from build123d import *

# Parameters (mm, degrees)
F0_R     = 3.5
F0_R_2   = 1.925
F1_DEPTH = 3.9
F2_DEPTH = 10
F4_DEPTH = 2
F5_R     = 0.25


with BuildPart() as f1:
    # F0 (on Front) → F1 (new body)
    with BuildSketch(Plane.XZ):
        Circle(F0_R)
        Circle(F0_R_2, mode=Mode.SUBTRACT)
        Circle(F0_R_2)
    extrude(amount=F1_DEPTH)

    # F0 (on Front) → F2 (join)
    with BuildSketch(Plane.XZ):
        Circle(F0_R_2)
    extrude(amount=-F2_DEPTH)

    # F3 (on face) → F4 (cut)
    with BuildSketch(Plane.XZ.offset(3.9)):
        Polygon((1.5, -0.8660254038), (1.5, 0.8660254038), (0, 1.7320508076), (-1.5, 0.8660254038), (-1.5, -0.8660254038), (0, -1.7320508076), align=None)
    extrude(amount=-F4_DEPTH, mode=Mode.SUBTRACT)

    # F5
    f5_edges = [f1.edges().sort_by_distance(p)[0] for p in [
        (-3.5, -3.9, 0),
    ]]
    fillet(f5_edges, radius=F5_R)


solid = f1.part
Read the model definition and answer for the solid it produces. Units are mm, in the model's axes. A direction names the side the tool comes from. Give positions to 0.01 mm unless a question says otherwise; leave off trailing zeros. Write each loop counter-clockwise with the first axis right and the second up, starting at its lowest first coordinate (ties: lowest second). Pieces come first, ordered by that corner, then holes. Notation, with made-up numbers: (66.5, -15) - (115.5, -15) arc R27 cw to (115.5, 23) - close; hole circle Ø7 at (-33.75, -31). An arc over 180 degrees is marked (long way). Answer in a Markdown table with one row per item. Add a question column.
Item 1: Section B-B, the plane z = 0 is taken. Write down the section's boundary in (x, y) (3 decimals).
Item 2: Section A-A, the plane y = -2.5 is taken. Write down the section's boundary in (x, z), and give its area (3 significant figures).
Item 3: A tool of negligible diameter and unlimited length cuts with its end or side. For faces 1 (the face through (-0.8, -3.9, 1.5)), 2 (the face through (2, 0, -2)), 3 (the face through (0, -1.9, 0)), from which of +Z, -Z, +X, -X, +Y, -Y can it reach the whole face along a straight path? Write none if from no direction.
Item 4: Flat-ended cylindrical pins translate along their axes: P1, Ø4, axis at x = -1, y = -2, coming from the +Z side; P2, Ø1.5, axis at x = -0.5, z = -0.5, coming from the -Y side; P3, Ø0.5, axis at y = -3, z = 0.5, coming from the +X side; P4, Ø2, axis at y = -1.5, z = 2, coming from the -X side. Find the tip coordinate at first contact, or state that the pin passes through.
Item 5: Section C-C, the plane y = 4 is taken. Write down the section's boundary in (x, z) (3 decimals).
Item 6: Find the intervals of material crossed by L1, parallel to Y at x = -1, z = 3; L2, parallel to Y at x = -1, z = -0.25; L3, parallel to X at y = -1.25, z = 1, in increasing order.
Item 7: Determine the mould class of faces 4 (the face through (0, 10, 0)), 5 (the face through (0.76, -2.914, 1.293)), 6 (the face through (3.233, -1.799, -1.341)) for opening direction X: pulls with the +X half, pulls with the -X half, needs draft (parallel to the pull), parting line crosses it, or undercut.
Recorded:
| question | item | result |
|---|---|---|
| 1 | outline | (-3.5, -3.65) arc R0.25 ccw to (-3.25, -3.9) - (-1.5, -3.9) - (-1.5, -1.9) - (1.5, -1.9) - (1.5, -3.9) - (3.25, -3.9) arc R0.25 ccw to (3.5, -3.65) - (3.5, 0) - (1.925, 0) - (1.925, 10) - (-1.925, 10) - (-1.925, 0) - (-3.5, 0) - close |
| 2 | outline | circle Ø7 at (0, 0); hole (-1.5, -0.87) - (0, -1.73) - (1.5, -0.87) - (1.5, 0.87) - (0, 1.73) - (-1.5, 0.87) - close |
| 2 | area | 30.7 mm2 |
| 3 | face 1 | +Z, -Z, +X, -X, -Y |
| 3 | face 2 | +Y |
| 3 | face 3 | -Y |
| 4 | P1 | stops at z = 3.5 |
| 4 | P2 | stops at y = -1.9 |
| 4 | P3 | stops at x = 3.49 |
| 4 | P4 | stops at x = -3.35 |
| 5 | outline | circle Ø3.85 at (0, 0) |
| 6 | L1 | y = -3.9 to 0 |
| 6 | L2 | y = -1.9 to 10 |
| 6 | L3 | x = -3.35 to 3.35 |
| 7 | face 4 | needs draft |
| 7 | face 5 | undercut |
| 7 | face 6 | parting line crosses it |
